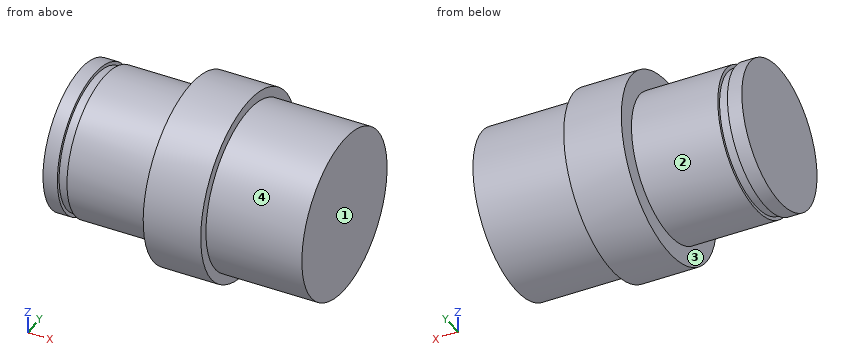
from build123d import *

# Parameters (mm, degrees)
ESBO_O2_W = 1
ESBO_O2_H = 0.35


with BuildPart() as part:
    # Esboço1 → Revolução1 (revolve)
    with BuildSketch(Plane.XY, mode=Mode.PRIVATE) as revolu_o1_sk:
        Polygon((0, 0), (0, 7.5), (11.5, 7.5), (11.5, 9.525), (17.5, 9.525), (17.5, 8.5), (27.5, 8.5), (27.5, 0), align=None)
    revolve(revolu_o1_sk.sketch.rotate(Axis((0, 0, 0), (1, 0, 0)), 90), axis=Axis((0, 0, 0), (1, 0, 0)))

    # Esboço2 → Corte-Revolução1 (revolve, cut)
    with BuildSketch(Plane.XY, mode=Mode.PRIVATE) as corte_revolu_o1_sk:
        with Locations((2, 7.325)):
            Rectangle(ESBO_O2_W, ESBO_O2_H)
    revolve(corte_revolu_o1_sk.sketch.rotate(Axis((0, 0, 0), (1, 0, 0)), 90), axis=Axis((0, 0, 0), (1, 0, 0)), mode=Mode.SUBTRACT)


solid = part.part
The listing builds one solid part. Answer for the finished solid, in the listing's coordinates (mm). Face numbers are marked on the shaded views. A direction names the side the tool comes from. Coordinates: 2 decimals unless noted, no trailing zeros. Write each loop counter-clockwise with the first axis right and the second up, starting at its lowest first coordinate (ties: lowest second). Pieces come first, ordered by that corner, then holes. Notation, with made-up numbers: M 45,7 L 52,7 A12 ccw 52,14 Z; hole C 88.25,26 d1. An arc over 180 degrees is marked long. Put each result on its own line as item: value. Start each with the question number.
1. A cutting plane is placed at D-D on x = 8. Write down the section's boundary in (y, z).
2. Flat-ended cylindrical pins translate along their axes: P1, Ø4, axis at x = 10, z = 4, coming from the +Y side; P2, Ø2, axis at x = 5, z = -2.5, coming from the -Y side; P3, Ø4, axis at x = 11, z = 6, coming from the -Y side. Find the tip coordinate at first contact, or state that the pin passes through.
3. A cutting plane is placed at C-C on x = 24.75. Write down the section's boundary in (y, z).
4. Consider line 1 (X direction, y = -4.25, z = 6); line 2 (Z direction, x = 2, y = 0.25); line 3 (X direction, y = 5.75, z = 6). Determine where each line is inside the solid, lowest interval first. Write a range as from..to.
5. Which of the six approach directions +Z, -Z, +X, -X, +Y, -Y give full straight-line access (tool end or side, diameter ignored) to the marked faces 1 and 2?
6. For a pull along Z with two mould halves and no side action, classify the marked faces 3 and 4 as pulls with the +Z half, pulls with the -Z half, needs draft (parallel to the pull), parting line crosses it, or undercut.
7. A cutting plane is placed at A-A on z = 0. Write down the section's boundary in (x, y) (3 decimals), then the cut area to 3 significant figures.
Resolved:
1. outline: C 0,0 d15
2. P1: stops at y = 9.14
2. P2: stops at y = -7.35
2. P3: stops at y = -8.61
3. outline: C 0,0 d17
4. line 1: x = 0..1.5, 2.5..27.5
4. line 2: z = -7.15..7.15
4. line 3: x = 11.5..27.5
5. face 1: +Z, -Z, +X, +Y, -Y
5. face 2: -X
6. face 3: needs draft
6. face 4: parting line crosses it
7. outline: M 0,-7.5 L 1.5,-7.5 L 1.5,-7.15 L 2.5,-7.15 L 2.5,-7.5 L 11.5,-7.5 L 11.5,-9.525 L 17.5,-9.525 L 17.5,-8.5 L 27.5,-8.5 L 27.5,8.5 L 17.5,8.5 L 17.5,9.525 L 11.5,9.525 L 11.5,7.5 L 2.5,7.5 L 2.5,7.15 L 1.5,7.15 L 1.5,7.5 L 0,7.5 Z
7. area: 456 mm2
